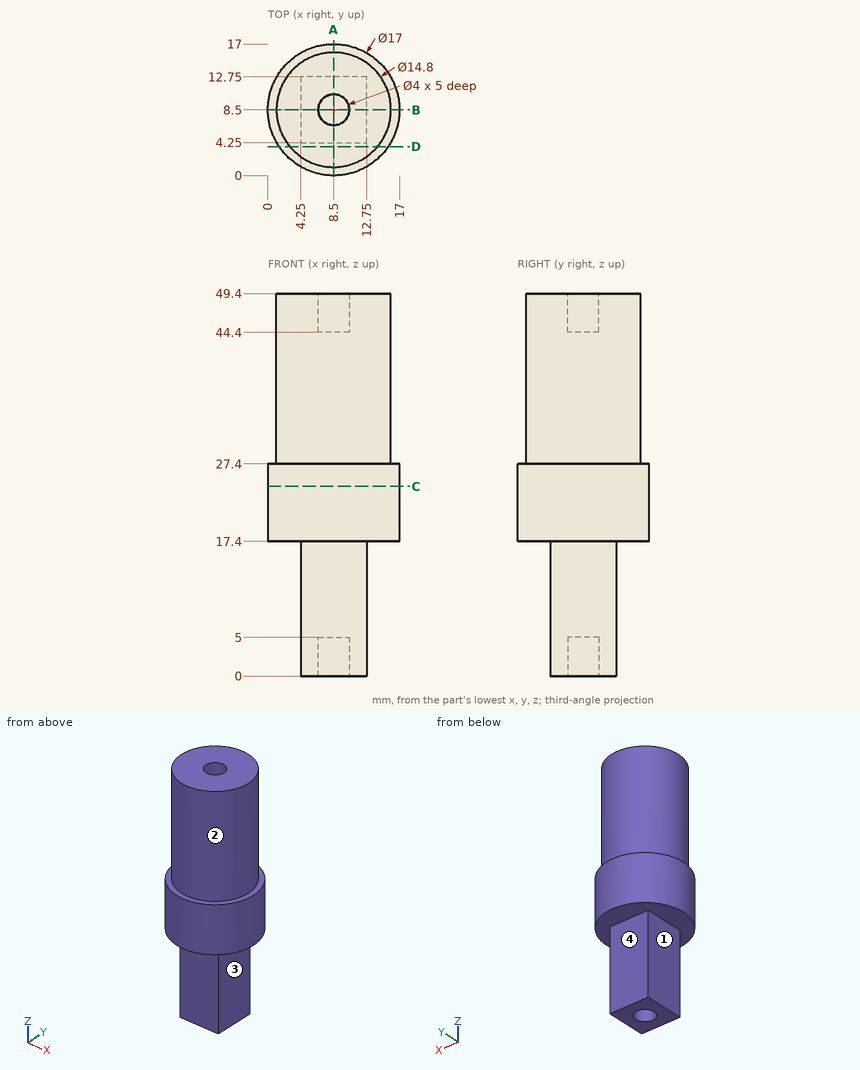
Study the drawing (mm; zero at the part's minimum x, y, z) and answer. A direction names the side the tool comes from. Give positions to 0.01 mm unless a question says otherwise; leave off trailing zeros. Loops run counter-clockwise (first coordinate to the right, second up) from the corner with the lowest first, then second, coordinate; pieces in that order, holes last. Notation, with made-up numbers: (12.5, -14) -> (58.5, -14) arc R27 cw to (58.5, 18) -> close; hole circle Ø5 at (89.5, -37). An arc over 180 degrees is marked (long way). Use a Markdown table: item, result. Add a question column.
1) The part is cut by section D-D, the plane y = 3.75. Determine the outline of the cut face in (x, z), plus the area to 3 significant figures.
2) The part is cut by section A-A, the plane x = 8.5. Determine the outline of the cut face in (y, z).
3) Consider line 1 along Y through (x, z) = (8.5, 46.05); line 2 along Z through (x, y) = (1, 8.5); line 3 along Y through (x, z) = (8.5, 3.1). Determine where each line is inside the solid, lowest interval first.
4) Each of these flat-tipped pins is pushed along its axis until it touches: P1, Ø2.5, axis at x = 8.5, y = 8.5, coming from the +Z side; P2, Ø4, axis at y = 8, z = 9.5, coming from the +X side; P3, Ø2, axis at y = 7.5, z = 12, coming from the -X side. Where does it stop, or does it pass through?
5) The part is cut by section C-C, the plane z = 24.5. Determine the outline of the cut face in (x, y).
6) Which of the six approach directions +Z, -Z, +X, -X, +Y, -Y give full straight-line access (tool end or side, diameter ignored) to the marked faces 1, 2, 3 and 4?
Reported:
| question | item | result |
|---|---|---|
| 1 | outline | (1.45, 17.4) -> (15.55, 17.4) -> (15.55, 27.4) -> (14.17, 27.4) -> (14.17, 49.4) -> (2.83, 49.4) -> (2.83, 27.4) -> (1.45, 27.4) -> close |
| 1 | area | 391 mm^2 |
| 2 | outline | (0, 17.4) -> (4.25, 17.4) -> (4.25, 0) -> (6.5, 0) -> (6.5, 5) -> (10.5, 5) -> (10.5, 0) -> (12.75, 0) -> (12.75, 17.4) -> (17, 17.4) -> (17, 27.4) -> (15.9, 27.4) -> (15.9, 49.4) -> (10.5, 49.4) -> (10.5, 44.4) -> (6.5, 44.4) -> (6.5, 49.4) -> (1.1, 49.4) -> (1.1, 27.4) -> (0, 27.4) -> close |
| 3 | line 1 | y = 1.1 to 6.5, 10.5 to 15.9 |
| 3 | line 2 | z = 17.4 to 27.4 |
| 3 | line 3 | y = 4.25 to 6.5, 10.5 to 12.75 |
| 4 | P1 | stops at z = 44.4 |
| 4 | P2 | stops at x = 12.75 |
| 4 | P3 | stops at x = 4.25 |
| 5 | outline | circle Ø17 at (8.5, 8.5) |
| 6 | face 1 | -Z, -X, +Y, -Y |
| 6 | face 2 | +Z |
| 6 | face 3 | -Z, +X, +Y, -Y |
| 6 | face 4 | -Z, +X, -X, +Y |
